Verification items for the finished model (mm, model axes). Give positions to 0.01 mm unless a question says otherwise; leave off trailing zeros. Order: outer loops, then holes, each group sorted by start corner. A loop starts at its lowest first (then second) coordinate and runs counter-clockwise, first axis right, second up. Notation, with made-up numbers: (54, 31) - (58, 31) arc R37 ccw to (58, 67) - close; hole circle Ø7 at (-37.75, -29.5). An arc over 180 degrees is marked (long way). Answer as a JSON object with one key per item and string values. Group by question number.
(1) Depth check by flat-ended pin: pin 1 Ø1 at (x, z) = (1, 161.5) entering from +Y; pin 2 Ø1.5 at (x, z) = (6.5, 152.5) entering from +Y; pin 3 Ø0.6 at (x, z) = (4.5, 1) entering from +Y. Enter the tip coordinate at first touch or a pass-through.
(2) Thickness scan on line 1 (Z direction, x = 5.75, y = -302.5); line 2 (Y direction, x = 9.5, z = 66); line 3 (Z direction, x = 5, y = -38). Record the ranges inside material, lowest first.
(3) Section check C-C (y = -31.5). Record the boundary of the cut face in (x, z), then the cut area to 3 significant figures.
(4) Section check B-B (z = 158.5). Record the boundary of the cut face in (x, y), then the cut area to 3 significant figures.
(5) Section check A-A (x = 8.5). Record the boundary of the cut face in (y, z).
```python
from build123d import *

# Parameters (mm, degrees)
F1_DEPTH = 10
F2_W     = 288.033763
F2_H     = 5
F3_DEPTH = 10.001
F4_R     = 3
F5_R     = 5
F7_DEPTH = 25


with BuildPart() as f1:
    # F0 (on Right) → F1 (new body)
    with BuildSketch(Plane.YZ):
        Polygon((-343.243208, 29.544233), (-338.033763, 0), (0, 0), (7.660444, 196.917872), (0, 203.345748), (-128.557522, 50.136859), (-330.443111, 14.538983), (-333.39513, 31.280714), align=None)
    extrude(amount=F1_DEPTH)

    # F2 (on face) → F3 (cut, through all)
    with BuildSketch(Plane.YZ.offset(10)):
        with Locations((-169.016881, 2.5)):
            Rectangle(F2_W, F2_H)
    extrude(amount=-F3_DEPTH, mode=Mode.SUBTRACT)

    # F4
    f4_edges = [f1.edges().sort_by_distance(p)[0] for p in [
        (5, 0, 203.345748),
        (5, 7.660444, 196.917872),
        (5, -25, 5),
        (5, -313.033763, 5),
        (5, -333.39513, 31.280714),
        (5, -343.243208, 29.544233),
    ]]
    fillet(f4_edges, radius=F4_R)

    # F5
    f5_edges = [f1.edges().sort_by_distance(p)[0] for p in [
        (5, -330.443111, 14.538983),
        (5, -128.557522, 50.136859),
    ]]
    fillet(f5_edges, radius=F5_R)

    # F6 (on face) → F7 (cut)
    with BuildSketch(Plane.YZ.offset(10)):
        with BuildLine():
            Line((-336.349554, 36.51854), (-333.280968, 19.115725))
            ThreePointArc((-333.280968, 19.115725), (-330.402348, 14.597198), (-325.171776, 13.437608))
            Line((-325.171776, 13.437608), (-130.002429, 47.85123))
            ThreePointArc((-130.002429, 47.85123), (-127.717966, 48.682706), (-125.855655, 50.245371))
            Line((-125.855655, 50.245371), (5.131385, 206.349646))
            Line((5.131385, 206.349646), (-336.349554, 36.51854))
        make_face()
    extrude(amount=-F7_DEPTH, mode=Mode.SUBTRACT)


solid = f1.part
```
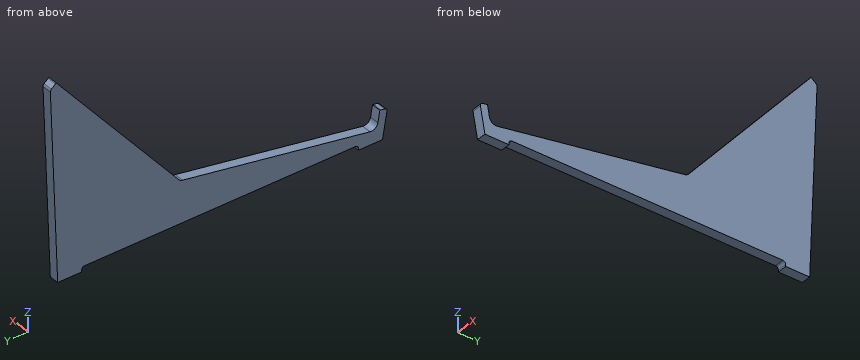
Solutions:
{
 "1": {"pin 1": "stops at y = 6.3", "pin 2": "stops at y = 5.96", "pin 3": "stops at y = 0.05"},
 "2": {"line 1": "z = 5 to 17.44", "line 2": "y = -112.64 to 2.57", "line 3": "z = 5 to 154.95"},
 "3": {"outline": "(0, 5) - (10, 5) - (10, 162.69) - (0, 162.69) - close", "area": "1,580 mm2"},
 "4": {"outline": "(0, -35.02) - (10, -35.02) - (10, 6.17) - (0, 6.17) - close", "area": "412 mm2"},
 "5": {"outline": "(-342.72, 26.59) - (-338.03, 0) - (-313.03, 0) - (-313.03, 2) arc R3 cw to (-310.03, 5) - (-28, 5) arc R3 cw to (-25, 2) - (-25, 0) - (0, 0) - (7.6, 195.45) arc R3 ccw to (6.53, 197.86) - (2.3, 201.42) arc R3 ccw to (1.42, 201.93) - (-125.86, 50.25) arc R7 cw to (-130, 47.85) - (-325.17, 13.44) arc R7 cw to (-333.28, 19.12) - (-335.33, 30.76) arc R3 ccw to (-336.35, 30.76) - (-340.29, 30.07) arc R3 ccw to start"}
}
